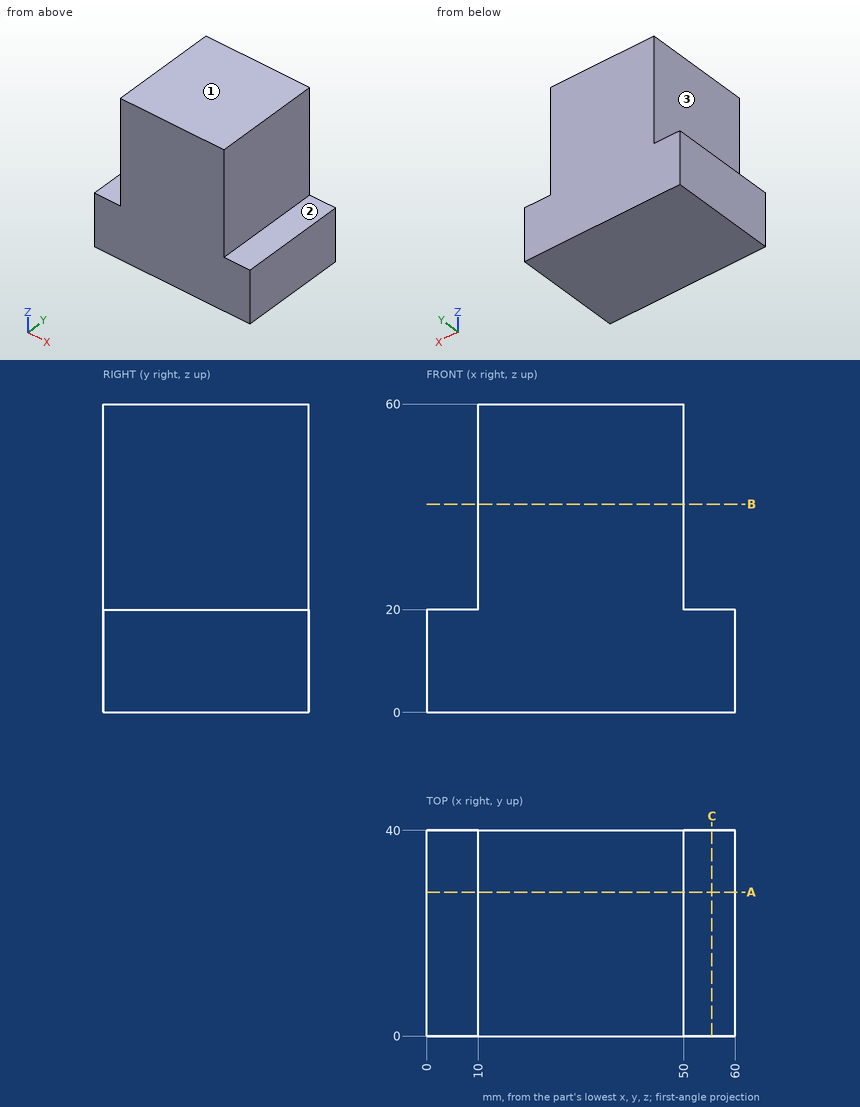
Check sheet for the drawn part. Datum: minimum x, y, z corner. Units: mm. A direction names the side the tool comes from. Round coordinates to 2 decimals unless told otherwise and drop trailing zeros. Loops run counter-clockwise (first coordinate to the right, second up) from the corner with the lowest first, then second, coordinate; pieces in that order, holes last. Notation, with made-up numbers: (-31.5, -18.75) - (2.5, -18.75) arc R24 ccw to (2.5, -6.75) - close; hole circle Ø6 at (61, 61.25). An arc over 180 degrees is marked (long way). Answer as a JSON object with one key per item and string values. Group by question number.
Q1. Sectioned sample at C-C, the plane x = 55.5. Enter the section's corners in (y, z).
Q2. Gauge pin test, flat ends, axial feed: P1, Ø20, axis at y = 25, z = 48, coming from the +X side; P2, Ø8, axis at x = 56, y = 20, coming from the +Z side; P3, Ø1, axis at y = 26, z = 53, coming from the -X side. Record the tip position at first contact, or that the pin passes through.
Q3. Scan lines: line 1 along Z through (x, y) = (5, 18); line 2 along X through (y, z) = (30.5, 57). Record each from-to range of solid material in increasing order. Write a range as [from, to].
Q4. Sectioned sample at B-B, the plane z = 40.5. Enter the section's corners in (x, y).
Q5. Set-up check for the marked faces 1, 2 and 3: record each of +Z, -Z, +X, -X, +Y, -Y from which the full face is reachable in a straight line by a thin tool's end or side.
Q6. Sectioned sample at A-A, the plane y = 28. Enter the section's corners in (x, z).
Solution:
{
 "1": {"outline": "(0, 0) - (40, 0) - (40, 20) - (0, 20) - close"},
 "2": {"P1": "stops at x = 50", "P2": "stops at z = 20", "P3": "stops at x = 10"},
 "3": {"line 1": "z = [0, 20]", "line 2": "x = [10, 50]"},
 "4": {"outline": "(10, 0) - (50, 0) - (50, 40) - (10, 40) - close"},
 "5": {"face 1": "+Z, +X, -X, +Y, -Y", "face 2": "+Z, +X, +Y, -Y", "face 3": "+Z, -X, +Y, -Y"},
 "6": {"outline": "(0, 0) - (60, 0) - (60, 20) - (50, 20) - (50, 60) - (10, 60) - (10, 20) - (0, 20) - close"}
}
